Part model, mm, in its own coordinate system. A direction names the side the tool comes from. Give positions to 0.01 mm unless a question says otherwise; leave off trailing zeros. Loops run counter-clockwise (first coordinate to the right, second up) from the corner with the lowest first, then second, coordinate; pieces in that order, holes last. Notation, with made-up numbers: (53, 30) -> (85, 30) arc R11 cw to (85, 42) -> close; hole circle Ø5 at (51, 19.25). An arc over 180 degrees is marked (long way). One line per question, with ' | ' between items.
```python
from build123d import *

# Parameters (mm, degrees)
SKETCH2_W                            = 16
SKETCH2_H                            = 38.1
BOSS_EXTRUDE1_DEPTH                  = 173.482
CONVERT_SOLID1_START                 = -173.482
CONVERT_SOLID1_DEPTH                 = 346.964
EDGE_FLANGE2_STRIP_W                 = 6.4008
EDGE_FLANGE2_STRIP_H                 = 1.2192
EDGE_FLANGE2_STRIP_CUT_DEPTH         = 346.964
EDGE_FLANGE2_DEPTH                   = 346.964
EDGE_FLANGE3_STRIP_W                 = 6.4008
EDGE_FLANGE3_STRIP_H                 = 1.2192
EDGE_FLANGE3_STRIP_CUT_DEPTH         = 172.6946
EDGE_FLANGE3_RELIEF_W                = 7.1628
EDGE_FLANGE3_RELIEF_H                = 1.6002
EDGE_FLANGE3_RELIEF_CUT_DEPTH        = 1.2192
EDGE_FLANGE3_DEPTH                   = 172.6946
PEM_CLEARANCE_HOLES_R                = 2.3876
CUT_EXTRUDE4_DEPTH                   = 179.335678775
TOP_PLATE_ATTACHMENT_PEM_HOLES_R     = 2.1082
CUT_EXTRUDE5_DEPTH                   = 179.335678775
CHAMFER2_SIZE                        = 8
SKETCH17_W                           = 20.9804
SKETCH17_H                           = 12.1158
CUT_EXTRUDE7_DEPTH                   = 1.2192
EDGE_FLANGE4_STRIP_W                 = 6.4008
EDGE_FLANGE4_STRIP_H                 = 1.2192
EDGE_FLANGE4_STRIP_CUT_DEPTH         = 17.78
EDGE_FLANGE4_RELIEF_W                = 7.1628
EDGE_FLANGE4_RELIEF_H                = 1.6002
EDGE_FLANGE4_RELIEF_CUT_DEPTH        = 1.2192
EDGE_FLANGE4_STRIP_2_W               = 6.4008
EDGE_FLANGE4_STRIP_2_H               = 1.2192
EDGE_FLANGE4_STRIP_CUT_2_DEPTH       = 17.78
EDGE_FLANGE4_RELIEF_2_W              = 7.1628
EDGE_FLANGE4_RELIEF_2_H              = 1.6002
EDGE_FLANGE4_RELIEF_CUT_2_DEPTH      = 1.2192
EDGE_FLANGE4_DEPTH                   = 17.78
EDGE_FLANGE4_BEND_DEPTH              = 17.78
BASE_MOUNTING_RIVET_CLAMPING_HOLES_R = 1.6637
CUT_EXTRUDE8_DEPTH                   = 1.2192
SKETCH29_R                           = 1.905
CUT_EXTRUDE11_DEPTH                  = 179.335678775
CHAMFER3_SIZE                        = 1.016


# Read off the part's stored shape, not the designer's step: Convert-Solid1
# Sheet-metal steps are written as plain solids
with BuildPart() as part:
    # Sketch2 → Boss-Extrude1 (new, symmetric)
    with BuildSketch(Plane.XY):
        with Locations((8, 19.05)):
            Rectangle(SKETCH2_W, SKETCH2_H)
    extrude(amount=BOSS_EXTRUDE1_DEPTH, both=True)

    # Convert-Solid1 outline → Convert-Solid1 (cut)
    with BuildSketch(Plane.XY.offset(CONVERT_SOLID1_START)):
        with BuildLine():
            Line((0, 38.1), (0, 36.1188))
            ThreePointArc((0, 36.1188), (0.580280045, 37.519719955), (1.9812, 38.1))
            Line((1.9812, 38.1), (0, 38.1))
        make_face()
        with BuildLine():
            Line((1.2192, 36.1188), (1.2192, 0))
            Line((1.2192, 0), (16, 0))
            Line((16, 0), (16, 36.8808))
            Line((16, 36.8808), (1.9812, 36.8808))
            ThreePointArc((1.9812, 36.8808), (1.442384633, 36.657615367), (1.2192, 36.1188))
        make_face()
    extrude(amount=CONVERT_SOLID1_DEPTH, mode=Mode.SUBTRACT)

    # Edge-Flange2 strip (across the edge) → Edge-Flange2 strip cut (cut)
    with BuildSketch(Plane(origin=(0, 0, -173.482), x_dir=(0, 1, 0), z_dir=(0, 0, 1))):
        with Locations((-1.2192, -0.6096)):
            Rectangle(EDGE_FLANGE2_STRIP_W, EDGE_FLANGE2_STRIP_H)
    extrude(amount=EDGE_FLANGE2_STRIP_CUT_DEPTH, mode=Mode.SUBTRACT)

    # Edge-Flange2 section (across the edge) → Edge-Flange2 (add)
    with BuildSketch(Plane(origin=(0, 0, -173.482), x_dir=(0, 1, 0), z_dir=(0, 0, 1))):
        with BuildLine():
            Line((0, 0.762), (0, 12.7508))
            Line((0, 12.7508), (1.2192, 12.7508))
            Line((1.2192, 12.7508), (1.2192, 0.762))
            ThreePointArc((1.2192, 0.762), (1.442384633, 0.223184633), (1.9812, 0))
            Line((1.9812, 0), (1.9812, -1.2192))
            ThreePointArc((1.9812, -1.2192), (0.580280045, -0.638919955), (0, 0.762))
        make_face()
    extrude(amount=EDGE_FLANGE2_DEPTH)

    # Edge-Flange3 strip (across the edge) → Edge-Flange3 strip cut (cut)
    with BuildSketch(Plane(origin=(-12.7508, 1.2192, -173.482), x_dir=(1, 0, 0), z_dir=(0, 0, 1))):
        with Locations((-1.2192, -0.6096)):
            Rectangle(EDGE_FLANGE3_STRIP_W, EDGE_FLANGE3_STRIP_H)
    extrude(amount=EDGE_FLANGE3_STRIP_CUT_DEPTH, mode=Mode.SUBTRACT)

    # Edge-Flange3 relief (on the sheet) → Edge-Flange3 relief cut (cut)
    with BuildSketch(Plane(origin=(-10.7696, 1.2192, -173.482), x_dir=(1, 0, 0), z_dir=(0, 1, 0))):
        with Locations((-2.8194, -173.4947)):
            Rectangle(EDGE_FLANGE3_RELIEF_W, EDGE_FLANGE3_RELIEF_H)
    extrude(amount=-EDGE_FLANGE3_RELIEF_CUT_DEPTH, mode=Mode.SUBTRACT)

    # Edge-Flange3 section (across the edge) → Edge-Flange3 (add)
    with BuildSketch(Plane(origin=(-12.7508, 1.2192, -173.482), x_dir=(1, 0, 0), z_dir=(0, 0, 1))):
        with BuildLine():
            Line((0, 0.762), (0, 5.6388))
            Line((0, 5.6388), (1.2192, 5.6388))
            Line((1.2192, 5.6388), (1.2192, 0.762))
            ThreePointArc((1.2192, 0.762), (1.442384633, 0.223184633), (1.9812, 0))
            Line((1.9812, 0), (1.9812, -1.2192))
            ThreePointArc((1.9812, -1.2192), (0.580280045, -0.638919955), (0, 0.762))
        make_face()
    extrude(amount=EDGE_FLANGE3_DEPTH)

    # PEM Clearance Holes → Cut-Extrude4 (cut, through all)
    with BuildSketch(Plane(origin=(0, 0, 0), x_dir=(1, 0, 0), z_dir=(0, 1, 0))):
        with Locations((-5.588, 22.098)):
            Circle(PEM_CLEARANCE_HOLES_R)
        with Locations((-5.588, 154.94)):
            Circle(PEM_CLEARANCE_HOLES_R)
        with Locations(Location((-5.588, -154.94, 0), (0, 0, 90))):
            Circle(PEM_CLEARANCE_HOLES_R)
        with Locations(Location((-5.588, -22.098, 0), (0, 0, 90))):
            Circle(PEM_CLEARANCE_HOLES_R)
    extrude(amount=CUT_EXTRUDE4_DEPTH, mode=Mode.SUBTRACT)

    # Top Plate Attachment PEM Holes → Cut-Extrude5 (cut, through all)
    with BuildSketch(Plane(origin=(0, 0, 0), x_dir=(1, 0, 0), z_dir=(0, 1, 0))):
        with Locations((8.89, -149.86)):
            Circle(TOP_PLATE_ATTACHMENT_PEM_HOLES_R)
        with Locations(Location((8.89, 149.86, 0), (0, 0, 90))):
            Circle(TOP_PLATE_ATTACHMENT_PEM_HOLES_R)
    extrude(amount=CUT_EXTRUDE5_DEPTH, mode=Mode.SUBTRACT)

    # Chamfer2
    chamfer2_edges = [part.edges().sort_by_distance(p)[0] for p in [
        (16, 37.4904, -173.482),
        (16, 37.4904, 173.482),
    ]]
    chamfer(chamfer2_edges, length=CHAMFER2_SIZE)

    # Sketch17 → Cut-Extrude7 (cut)
    with BuildSketch(Plane(origin=(0, 0, 0), x_dir=(0, 0, -1), z_dir=(1, 0, 0))):
        with Locations((-22.098, 23.1521)):
            Rectangle(SKETCH17_W, SKETCH17_H)
        with Locations((-154.94, 23.1521)):
            Rectangle(SKETCH17_W, SKETCH17_H)
    extrude(amount=CUT_EXTRUDE7_DEPTH, mode=Mode.SUBTRACT)

    # Edge-Flange4 strip (across the edge) → Edge-Flange4 strip cut (cut)
    with BuildSketch(Plane(origin=(0, 29.21, 13.208), x_dir=(0, 1, 0), z_dir=(0, 0, 1))):
        with Locations((-2.4384, -0.6096)):
            Rectangle(EDGE_FLANGE4_STRIP_W, EDGE_FLANGE4_STRIP_H)
    extrude(amount=EDGE_FLANGE4_STRIP_CUT_DEPTH, mode=Mode.SUBTRACT)

    # Edge-Flange4 relief (on the sheet) → Edge-Flange4 relief cut (cut)
    with BuildSketch(Plane(origin=(0, 29.972, 13.208), x_dir=(0, 1, 0), z_dir=(-1, 0, 0))):
        with Locations((-2.8194, 0.8001)):
            Rectangle(EDGE_FLANGE4_RELIEF_W, EDGE_FLANGE4_RELIEF_H)
        with Locations((-2.8194, -18.5801)):
            Rectangle(EDGE_FLANGE4_RELIEF_W, EDGE_FLANGE4_RELIEF_H)
    extrude(amount=-EDGE_FLANGE4_RELIEF_CUT_DEPTH, mode=Mode.SUBTRACT)

    # Edge-Flange4 strip 2 (across the edge) → Edge-Flange4 strip cut 2 (cut)
    with BuildSketch(Plane(origin=(0, 29.21, 146.05), x_dir=(0, 1, 0), z_dir=(0, 0, 1))):
        with Locations((-2.4384, -0.6096)):
            Rectangle(EDGE_FLANGE4_STRIP_2_W, EDGE_FLANGE4_STRIP_2_H)
    extrude(amount=EDGE_FLANGE4_STRIP_CUT_2_DEPTH, mode=Mode.SUBTRACT)

    # Edge-Flange4 relief 2 (on the sheet) → Edge-Flange4 relief cut 2 (cut)
    with BuildSketch(Plane(origin=(0, 29.972, 146.05), x_dir=(0, 1, 0), z_dir=(-1, 0, 0))):
        with Locations((-2.8194, 0.8001)):
            Rectangle(EDGE_FLANGE4_RELIEF_2_W, EDGE_FLANGE4_RELIEF_2_H)
        with Locations((-2.8194, -18.5801)):
            Rectangle(EDGE_FLANGE4_RELIEF_2_W, EDGE_FLANGE4_RELIEF_2_H)
    extrude(amount=-EDGE_FLANGE4_RELIEF_CUT_2_DEPTH, mode=Mode.SUBTRACT)

    # Edge-Flange4 section (across the edge) → Edge-Flange4 (add)
    with BuildSketch(Plane(origin=(0, 29.21, 13.208), x_dir=(0, 1, 0), z_dir=(0, 0, 1))):
        with BuildLine():
            Line((-1.2192, 0.762), (-1.2192, 10.2108))
            Line((-1.2192, 10.2108), (0, 10.2108))
            Line((0, 10.2108), (0, 0.762))
            ThreePointArc((0, 0.762), (0.223184633, 0.223184633), (0.762, 0))
            Line((0.762, 0), (0.762, -1.2192))
            ThreePointArc((0.762, -1.2192), (-0.638919955, -0.638919955), (-1.2192, 0.762))
        make_face()
    extrude(amount=EDGE_FLANGE4_DEPTH)

    # Edge-Flange4 section 2 (across the edge) → Edge-Flange4 bend (add)
    with BuildSketch(Plane(origin=(0, 29.21, 146.05), x_dir=(0, 1, 0), z_dir=(0, 0, 1))):
        with BuildLine():
            Line((-1.2192, 0.762), (-1.2192, 10.2108))
            Line((-1.2192, 10.2108), (0, 10.2108))
            Line((0, 10.2108), (0, 0.762))
            ThreePointArc((0, 0.762), (0.223184633, 0.223184633), (0.762, 0))
            Line((0.762, 0), (0.762, -1.2192))
            ThreePointArc((0.762, -1.2192), (-0.638919955, -0.638919955), (-1.2192, 0.762))
        make_face()
    extrude(amount=EDGE_FLANGE4_BEND_DEPTH)

    # Base Mounting Rivet Clamping Holes → Cut-Extrude8 (cut)
    with BuildSketch(Plane(origin=(0, 0, 0), x_dir=(1, 0, 0), z_dir=(0, 1, 0))):
        with Locations(Location((-5.588, -165.1, 0), (0, 0, 90))):
            Circle(BASE_MOUNTING_RIVET_CLAMPING_HOLES_R)
        with Locations(Location((-5.588, 0, 0), (0, 0, 270))):
            Circle(BASE_MOUNTING_RIVET_CLAMPING_HOLES_R)
        with Locations(Location((-5.588, 165.1, 0), (0, 0, 270))):
            Circle(BASE_MOUNTING_RIVET_CLAMPING_HOLES_R)
    extrude(amount=CUT_EXTRUDE8_DEPTH, mode=Mode.SUBTRACT)

    # Sketch29 → Cut-Extrude11 (cut, through all)
    with BuildSketch(Plane(origin=(0, 0, 0), x_dir=(1, 0, 0), z_dir=(0, 1, 0))):
        with Locations((-5.588, -22.098)):
            Circle(SKETCH29_R)
        with Locations(Location((-5.588, -154.94, 0), (0, 0, 180))):
            Circle(SKETCH29_R)
    extrude(amount=CUT_EXTRUDE11_DEPTH, mode=Mode.SUBTRACT)

    # Chamfer3
    chamfer3_edges = [part.edges().sort_by_distance(p)[0] for p in [
        (-10.2108, 28.6004, 13.208),
        (-10.2108, 28.6004, 30.988),
        (-10.2108, 28.6004, 146.05),
        (-10.2108, 28.6004, 163.83),
        (-12.7508, 0.6096, 173.482),
        (-12.7508, 0.6096, 0.8128),
        (-12.1412, 6.858, -173.482),
        (-12.1412, 6.858, -0.7874),
    ]]
    chamfer(chamfer3_edges, length=CHAMFER3_SIZE)


solid = part.part
```
1) Drill centre lines: line 1 (Y direction, x = -2.5, z = -146); line 2 (Y direction, x = 9.5, z = -6.5). Where is each one in solid material? Low to high.
Found:
line 1: 0 to 1.22 | line 2: 36.88 to 38.1
2) Saw through at A-A (z = -71.5). Give the cut face in (x, y).
Found:
outline: (-12.75, 1.98) arc R1.98 ccw to (-10.77, 0) -> (-0.76, 0) arc R1.98 ccw to (1.22, 1.98) -> (1.22, 36.12) arc R0.76 cw to (1.98, 36.88) -> (16, 36.88) -> (16, 38.1) -> (1.98, 38.1) arc R1.98 ccw to (0, 36.12) -> (0, 1.98) arc R0.76 cw to (-0.76, 1.22) -> (-10.77, 1.22) arc R0.76 cw to (-11.53, 1.98) -> (-11.53, 6.86) -> (-12.75, 6.86) -> close
3) Tool access for faces 1 (the flat face through (12.056, 37.482, -169.426)), 2 (the flat face through (1.219, 19, -2)), 3 (the flat face through (-6, 29.21, 20)): list every direction of +Z, -Z, +X, -X, +Y, -Y with a clear straight run to the whole face (end or side of a thin tool).
Found:
face 1: -Z, +X, +Y, -Y | face 2: +Z, -Z, +X, -Y | face 3: +Z, -Z, -X, +Y
4) Pin check, flat tips, straight feed: P1, Ø8, axis at x = -0.5, z = -79.5, coming from the +Y side; P2, Ø12, axis at y = 8, z = -47.5, coming from the +X side; P3, Ø6, axis at x = -5, z = 67.5, coming from the +Y side; P4, Ø4.5, axis at x = -5.588, z = 154.94, coming from the +Y side. Stop position of each tip, or through.
Found:
P1: y = 38.1 | P2: x = 1.22 | P3: y = 1.22 | P4: y = 29.21
5) Pull direction Y, two halves, no side cores. Call faces 4 (the flat face through (11.94, 37.48, 169.54)), 5 (the flat face through (-5, 27.991, 20)), 6 (the flat face through (-5.4, 27.991, 152.8)), 7 (the flat face through (-7, 0, -2)): pulls with the +Y half, pulls with the -Y half, needs draft (parallel to the pull), parting line crosses it, or undercut.
Found:
face 4: needs draft | face 5: undercut | face 6: undercut | face 7: pulls with the -Y half
